For this review, use the dimensioned drawing (mm, ordinates from the lowest corner) and the shaded views. A direction names the side the tool comes from. Round coordinates to 2 decimals unless told otherwise and drop trailing zeros. Loops run counter-clockwise (first coordinate to the right, second up) from the corner with the lowest first, then second, coordinate; pieces in that order, holes last. Notation, with made-up numbers: (83, 43) -> (130, 43) arc R21 ccw to (130, 67) -> close; hole circle Ø5 at (68.25, -39.5). An arc over 180 degrees is marked (long way). Answer as CSV lines item,"result". Start each with the question number.
(1) Take a section at B-B, the plane x = 1. Write out the cut boundary in (y, z), and give its area (3 significant figures).
(2) Machinability: for the marked faces 1 and 2, which of the approach directions +Z, -Z, +X, -X, +Y, -Y give a long, thin tool a straight path to every point of the face, cutting with its end or side? Answer none if there is none.
(3) For P1, Ø1, axis at x = 1, z = 5.5, coming from the +Y side; P2, Ø1, axis at x = 0.5, y = 2, coming from the +Z side, all flat-tipped, find the tip position at first contact; note any pin that passes through.
(4) Take a section at A-A, the plane y = 1.6. Write out the cut boundary in (x, z).
(5) To check wall thickness, follow line 1 (Z direction, x = 1.75, y = 0.4); line 2 (X direction, y = 1.1, z = 6.25); line 3 (Z direction, x = 1.15, y = 0.6). State the ranges of each line that lie inside material, in increasing order. Write a range as from..to.
(6) Take a section at C-C, the plane z = 2.5. Write out the cut boundary in (x, y), and give its area (3 significant figures).
(7) Take a section at D-D, the plane y = 1. Write out the cut boundary in (x, z).
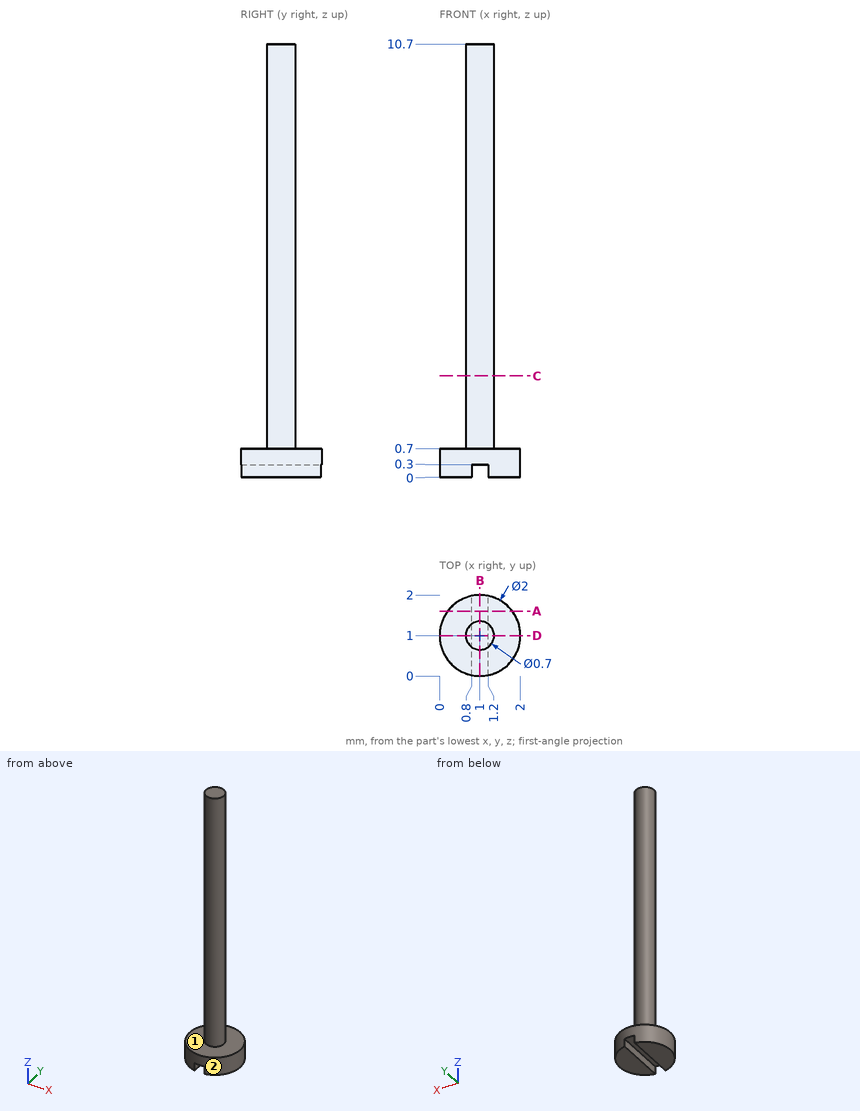
The answers:
1,outline,"(0, 0.3) -> (2, 0.3) -> (2, 0.7) -> (1.35, 0.7) -> (1.35, 10.7) -> (0.65, 10.7) -> (0.65, 0.7) -> (0, 0.7) -> close"
1,area,"7.80 mm²"
2,face 1,"+Z"
2,face 2,"+Z, -Z"
3,P1,"y = 1.35"
3,P2,"z = 0.7"
4,outline,"(0.2, 0) -> (0.8, 0) -> (0.8, 0.3) -> (1.2, 0.3) -> (1.2, 0) -> (1.8, 0) -> (1.8, 0.7) -> (0.2, 0.7) -> close"
5,line 1,"0..0.7"
5,line 2,"0.66..1.34"
5,line 3,"0.3..0.7"
6,outline,"circle Ø0.7 at (1, 1)"
6,area,"0.385 mm²"
7,outline,"(0, 0) -> (0.8, 0) -> (0.8, 0.3) -> (1.2, 0.3) -> (1.2, 0) -> (2, 0) -> (2, 0.7) -> (1.35, 0.7) -> (1.35, 10.7) -> (0.65, 10.7) -> (0.65, 0.7) -> (0, 0.7) -> close"
